Check sheet for the modelled part. Datum: model origin and axes. Units: mm. Face numbers are marked on the shaded views. A direction names the side the tool comes from. Round coordinates to 2 decimals unless told otherwise and drop trailing zeros. Write each loop counter-clockwise with the first axis right and the second up, starting at its lowest first coordinate (ties: lowest second). Pieces come first, ordered by that corner, then holes.
Item 1: Cross-section at A-A on x = 0. Enter the section's corners in (y, z), plus the area to 3 significant figures.
Item 2: Release check for a two-part mould opening along Y. For the marked faces 4, 5 and 6 record: +Y half, -Y half, draft (parallel to the pull), parting line (faces both ways), or undercut.
Item 3: Cross-section at D-D on z = 2.7. Enter the section's corners in (x, y), plus the area to 3 significant figures.
Item 4: Material ranges on line 1 (Y direction, x = 0, z = 2.1); line 2 (Z direction, x = -0.55, y = -12.5); line 3 (X direction, y = -12.25, z = 1.35), recorded low to high.
Item 5: Cross-section at B-B on z = 1.45. Enter the section's corners in (x, y).
Item 6: Tool access check on the marked faces 1, 2 and 3. Record the directions out of +Z, -Z, +X, -X, +Y, -Y that give a thin tool (end or side, any length) a straight path to the whole face; none if there is none.
Item 7: Go/stop test with flat-tipped pins: pin 1 Ø0.6 at (y, z) = (-10, 2) entering from +X; pin 2 Ø1 at (y, z) = (-3, 1) entering from -X; pin 3 Ø1.5 at (x, y) = (0.5, -12.5) entering from -Z; pin 4 Ø1.5 at (x, y) = (0, -2) entering from -Z. Record where each tip stops, or that it passes through.
Item 8: Cross-section at C-C on y = -5.5. Enter the section's corners in (x, z).
from build123d import *

# Parameters (mm, degrees)
SKETCH_1_R      = 2
SKETCH_1_R_2    = 1.5
EXTRUDE_1_DEPTH = 3
SKETCH_2_W      = 3
SKETCH_2_H      = 2
EXTRUDE_2_DEPTH = 15


with BuildPart() as part:
    # 草图1 → 凸台-拉伸1 (new body)
    with BuildSketch(Plane.XY):
        with BuildLine():
            ThreePointArc((0, -2), (-1.414213562, -1.414213562), (-2, 0))
            Line((-2, 0), (-2, -2))
            Line((-2, -2), (0, -2))
        make_face()
        Circle(SKETCH_1_R)
        Circle(SKETCH_1_R_2, mode=Mode.SUBTRACT)
        with BuildLine():
            Line((2, -2), (2, 0))
            ThreePointArc((2, 0), (1.414213562, -1.414213562), (0, -2))
            Line((0, -2), (2, -2))
        make_face()
    extrude(amount=EXTRUDE_1_DEPTH)

    # 草图2 → 凸台-拉伸2 (add)
    with BuildSketch(Plane.XZ.offset(2)):
        with Locations((0, 1.5)):
            Rectangle(SKETCH_2_W, SKETCH_2_H)
    extrude(amount=EXTRUDE_2_DEPTH)


solid = part.part
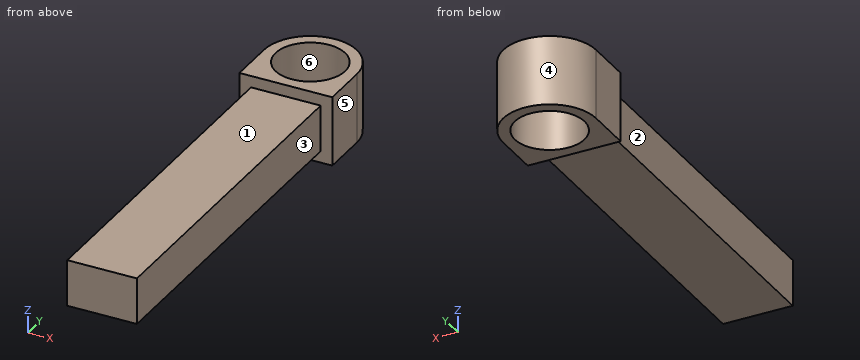
Response values:
1. outline: (-17, 0.5) - (-2, 0.5) - (-2, 0) - (-1.5, 0) - (-1.5, 3) - (-2, 3) - (-2, 2.5) - (-17, 2.5) - close; (1.5, 0) - (2, 0) - (2, 3) - (1.5, 3) - close
1. area: 33.0 mm2
2. face 4: +Y half
2. face 5: draft
2. face 6: undercut
3. outline: (-2, -2) - (2, -2) - (2, 0) arc R2 ccw to (-2, 0) - close; hole circle Ø3 at (0, 0)
3. area: 7.21 mm2
4. line 1: y = -17 to -1.5, 1.5 to 2
4. line 2: z = 0.5 to 2.5
4. line 3: x = -1.5 to 1.5
5. outline: (-2, -2) - (-1.5, -2) - (-1.5, -17) - (1.5, -17) - (1.5, -2) - (2, -2) - (2, 0) arc R2 ccw to (-2, 0) - close; hole circle Ø3 at (0, 0)
6. face 1: +Z, +X, -X, -Y
6. face 2: +Z, -Z, -X, -Y
6. face 3: +Z, -Z, +X, -Y
7. pin 1: stops at x = 1.5
7. pin 2: stops at x = -1.5
7. pin 3: stops at z = 0.5
7. pin 4: stops at z = 0
8. outline: (-1.5, 0.5) - (1.5, 0.5) - (1.5, 2.5) - (-1.5, 2.5) - close
